Job drawing, mm, ordinate dimensions from the low corner. One solid piece. A direction names the side the tool comes from. Coordinates: 2 decimals unless noted, no trailing zeros. Loops run counter-clockwise (first coordinate to the right, second up) from the corner with the lowest first, then second, coordinate; pieces in that order, holes last. Notation, with made-up numbers: (2, -40) -> (25, -40) arc R10 cw to (25, -34) -> close; hole circle Ø3 at (-1, 20). An arc over 180 degrees is marked (long way). Use one line per item in the form item = value. Start each with the question number.
(1) Mould opens along X. For the marked faces 5, 6 and 7 say: +X half, -X half, draft (parallel to the pull), parting line (faces both ways), or undercut.
(2) 3-axis set-ups, long thin cutter, end or side, ignore diameter. For the marked faces 1, 2, 3 and 4: which of +Z, -Z, +X, -X, +Y, -Y reach the whole face in a straight line?
(3) Band-saw the part on B-B on z = 39.5. Give the cut face in (x, y) (1 decimal), then the cut area to 3 significant figures.
(4) Band-saw the part on A-A on x = 10. Give the cut face in (y, z) (1 decimal), then the cut area to 3 significant figures.
(5) Drill centre lines: L1, parallel to Z at x = 10.5, y = 86.5 (1 decimal); L2, parallel to Z at x = 10, y = 77 (1 decimal); L3, parallel to X at y = 78, z = 32 (1 decimal). Where is each one in solid material? Low to high. Write a range as [from, to].
(6) Pin check, flat tips, straight feed: P1, Ø6, axis at x = 9.5, z = 16.5, coming from the -Y side; P2, Ø25, axis at y = 31, z = 24, coming from the -X side; P3, Ø6, axis at x = 12.5, z = 35, coming from the -Y side. Stop position of each tip, or through.
(7) Band-saw the part on D-D on x = 64.5. Give the cut face in (y, z).
(8) Band-saw the part on C-C on y = 37. Give the cut face in (x, z).
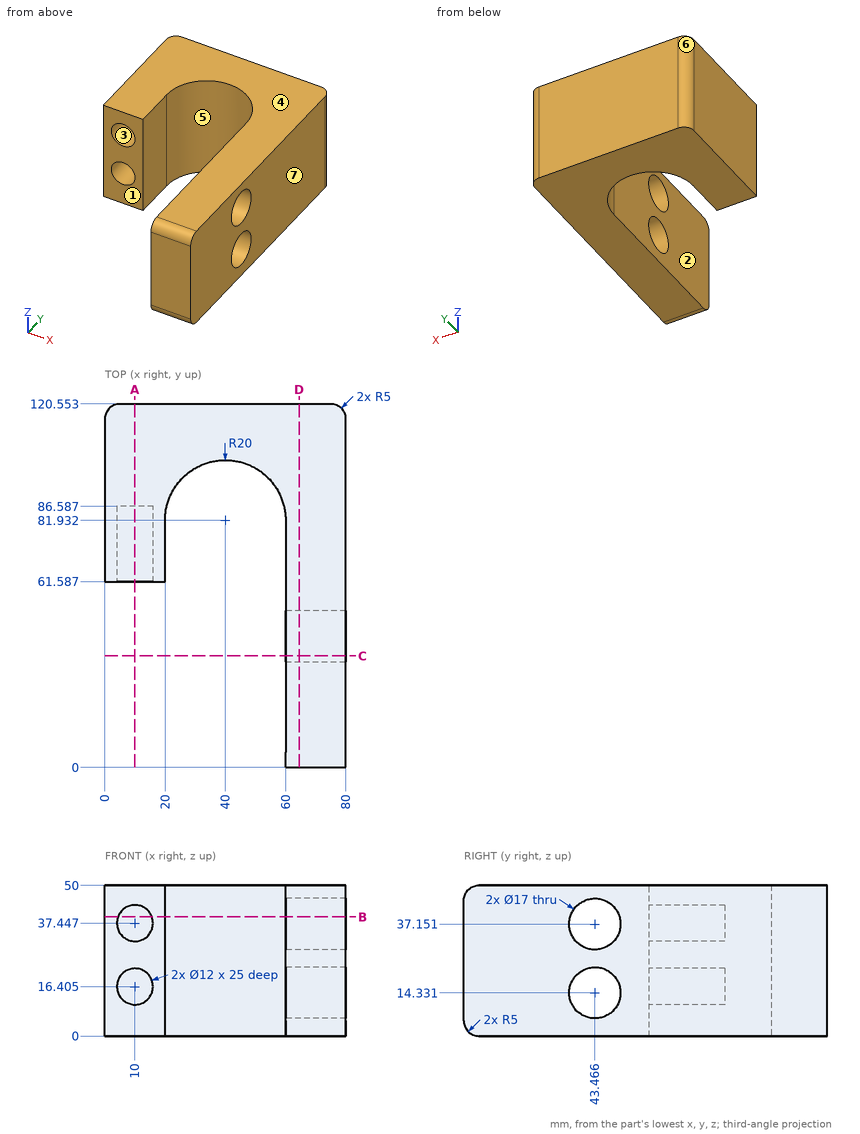
A:
q1.face_5 = undercut
q1.face_6 = -X half
q1.face_7 = +X half
q2.face_1 = +Z, -Z, -X, -Y
q2.face_2 = +Z, -Z, -Y
q2.face_3 = -Y
q2.face_4 = +Z, +X, -X, +Y, -Y
q3.outline = (0, 61.6) -> (4.4, 61.6) -> (4.4, 86.6) -> (15.6, 86.6) -> (15.6, 61.6) -> (20, 61.6) -> (20, 81.9) arc R20 cw to (60, 81.9) -> (60, 51.6) -> (80, 51.6) -> (80, 115.6) arc R5 ccw to (75, 120.6) -> (5, 120.6) arc R5 ccw to (0, 115.6) -> close; (60, 0) -> (80, 0) -> (80, 35.3) -> (60, 35.3) -> close
q3.area = 3,890 mm²
q4.outline = (61.6, 0) -> (120.6, 0) -> (120.6, 50) -> (61.6, 50) -> (61.6, 43.4) -> (86.6, 43.4) -> (86.6, 31.4) -> (61.6, 31.4) -> (61.6, 22.4) -> (86.6, 22.4) -> (86.6, 10.4) -> (61.6, 10.4) -> close
q4.area = 2,350 mm²
q5.L1 = [0, 10.4], [22.4, 31.5], [43.4, 50]
q5.L2 = [0, 10.4], [22.4, 31.4], [43.4, 50]
q5.L3 = [0, 7.5], [12.5, 20], [60, 80]
q6.P1 = 86.59
q6.P2 = 60
q6.P3 = 61.59
q7.outline = (0, 5) arc R5 ccw to (5, 0) -> (120.55, 0) -> (120.55, 50) -> (5, 50) arc R5 ccw to (0, 45) -> close; hole circle Ø17 at (43.47, 14.33); hole circle Ø17 at (43.47, 37.15)
q8.outline = (60, 0) -> (80, 0) -> (80, 8.81) -> (60, 8.81) -> close; (60, 19.85) -> (80, 19.85) -> (80, 31.63) -> (60, 31.63) -> close; (60, 42.67) -> (80, 42.67) -> (80, 50) -> (60, 50) -> close
